```python
from build123d import *

# Parameters (mm, degrees)
BOSS_EXTRUDE1_DEPTH                = 6.35
F_1_16_0_0625_DIAMETER_HOLE1_D     = 1.5875
F_1_16_0_0625_DIAMETER_HOLE1_DEPTH = 1.5875
F_1_16_0_0625_DIAMETER_HOLE1_TIP   = 0.476933116
F_3_32_0_09375_DIAMETER_HOLE1_D    = 2.38125


with BuildPart() as part:
    # Sketch1 → Boss-Extrude1 (new body)
    with BuildSketch(Plane(origin=(0, 0, 0), x_dir=(1, 0, 0), z_dir=(0, 1, 0))):
        with BuildLine():
            Line((6.814332014, 0), (10.9982, 0))
            Line((10.9982, 0), (10.9982, 6.35))
            Line((10.9982, 6.35), (0, 6.35))
            Line((0, 6.35), (0, 0))
            Line((0, 0), (4.183867986, 0))
            ThreePointArc((4.183867986, 0), (5.4991, 0.6985), (6.814332014, 0))
        make_face()
    extrude(amount=BOSS_EXTRUDE1_DEPTH)

    # 1/16 (0.0625) Diameter Hole1
    with Locations(Plane.XY):
        with Locations((2.3241, 3.175), (8.6741, 3.175)):
            Hole(F_1_16_0_0625_DIAMETER_HOLE1_D / 2, depth=F_1_16_0_0625_DIAMETER_HOLE1_DEPTH)
            with Locations((0, 0, -(F_1_16_0_0625_DIAMETER_HOLE1_DEPTH + F_1_16_0_0625_DIAMETER_HOLE1_TIP / 2))):  # 118° drill point
                Cone(0, F_1_16_0_0625_DIAMETER_HOLE1_D / 2, F_1_16_0_0625_DIAMETER_HOLE1_TIP, mode=Mode.SUBTRACT)

    # 3/32 (0.09375) Diameter Hole1 (through all)
    with Locations(Plane(origin=(10.9982, 0, 0), x_dir=(0, 0, -1), z_dir=(1, 0, 0))):
        with Locations((4.7625, 3.175)):
            Hole(F_3_32_0_09375_DIAMETER_HOLE1_D / 2)


solid = part.part
```
CAD build for the part. Positions are in the model's coordinates, mm. A direction names the side the tool comes from. Give positions to 0.01 mm unless a question says otherwise; leave off trailing zeros. Write each loop counter-clockwise with the first axis right and the second up, starting at its lowest first coordinate (ties: lowest second). Pieces come first, ordered by that corner, then holes. Notation, with made-up numbers: (50, 63.25) -> (95, 63.25) arc R28 cw to (95, 81.25) -> close; hole circle Ø5 at (83.5, 9.5). An arc over 180 degrees is marked (long way). Write each question's results on one line, items separated by ' | '.
1. Two-plate mould, pull along Z, no slides. Class faces 1 (the flat face through (5, 0, -3)), 2 (the flat face through (6, 3, -6.35)), 3 (the conical face through (8.8, 3.12, -1.98)), 4 (the cylindrical face through (5.422, 2.719, -3.663)): pulls with the +Z half, pulls with the -Z half, needs draft (parallel to the pull), parting line crosses it, or undercut.
Geometry check:
face 1: needs draft | face 2: pulls with the -Z half | face 3: pulls with the +Z half | face 4: undercut
2. Cut at A-A, the plane z = -4.5. Write the cut outline in (x, y).
Geometry check:
outline: (0, 0) -> (11, 0) -> (11, 2.01) -> (0, 2.01) -> close; (0, 4.34) -> (11, 4.34) -> (11, 6.35) -> (0, 6.35) -> close
3. Cut at C-C, the plane z = -0.5. Give the number of separate pieces and of enclosed holes in the cut face, then the cut area to 3 significant figures.
Geometry check:
separate pieces: 2 | enclosed holes: 2 | area: 56.1 mm²
4. Wall check: probe 1 along Z at (x, y) = (1, 3.25); probe 2 along X at (y, z) = (3, -0.5); probe 3 along Y at (x, z) = (9.5, -3.75). Give the ranges that are in metal, low to high. Write a range as [from, to].
Geometry check:
probe 1: [-6.35, -5.95], [-3.57, 0] | probe 2: [0, 1.55], [3.1, 4.73], [6.27, 7.9], [9.45, 11] | probe 3: [0, 2.55], [3.8, 6.35]
5. Which spindle directions (+Z, -Z, +X, -X, +Y, -Y) get a long thin tool onto all of the face, cutting with end or side? Do faces 5 (the cylindrical face through (7.94, 2.87, -0.8)), 6 (the flat face through (5, 6.35, -3)). Say none if no direction does.
Geometry check:
face 5: +Z | face 6: +Z, -Z, +X, -X, +Y
